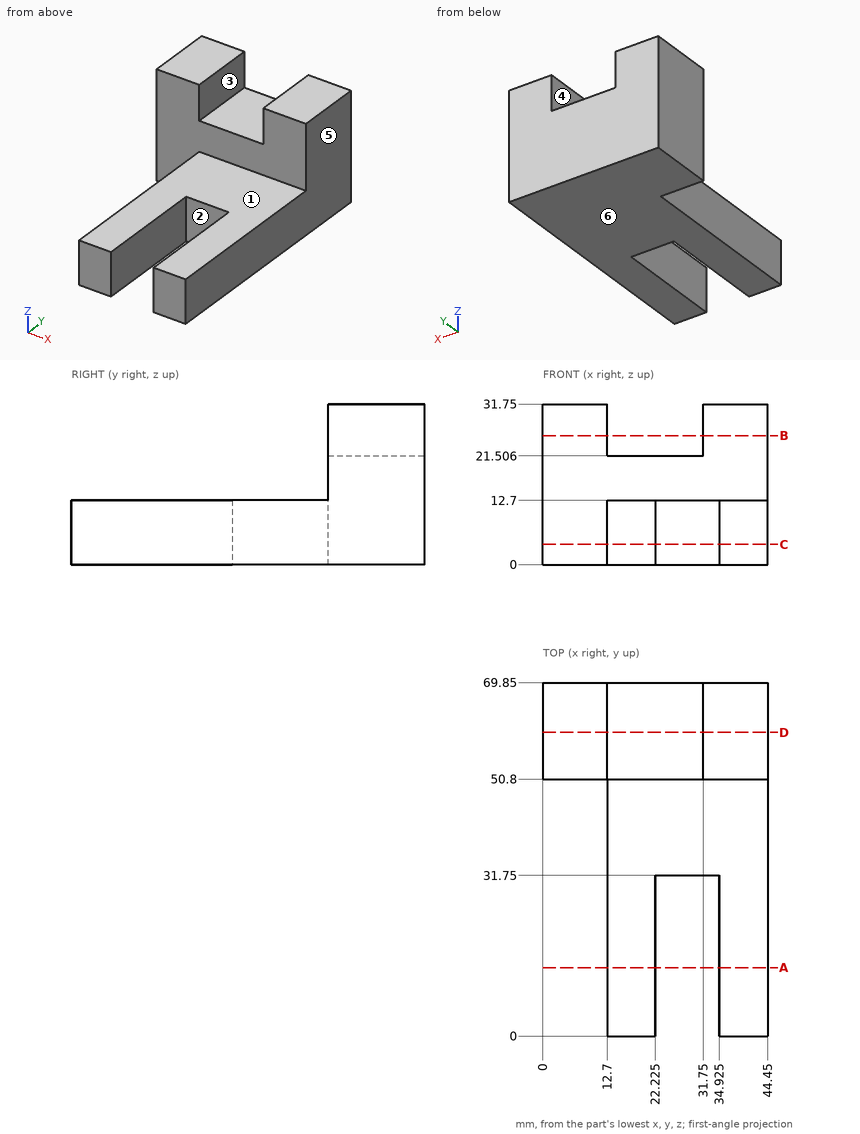
Print and shaded views of the part. All mm, measured from the part's lowest x, y and z. A direction names the side the tool comes from. Round coordinates to 2 decimals unless told otherwise and drop trailing zeros. Write each loop counter-clockwise with the first axis right and the second up, starting at its lowest first coordinate (ties: lowest second). Pieces come first, ordered by that corner, then holes. Notation, with made-up numbers: (55, 87.5) -> (110, 87.5) arc R10 ccw to (110, 106.5) -> close; hole circle Ø3 at (13, 3). An arc over 180 degrees is marked (long way). Answer in a Markdown table with one row per item. Add a question column.
Item 1: Saw through at D-D, the plane y = 60. Write the cut outline in (x, z).
Item 2: Saw through at A-A, the plane y = 13.5. Write the cut outline in (x, z) (3 decimals), then the cut area to 3 significant figures.
Item 3: Drop flat-ended pins along their axis: pin 1 Ø5 at (x, z) = (23, 20) entering from -Y; pin 2 Ø15 at (x, y) = (23, 65) entering from +Z; pin 3 Ø14 at (y, z) = (19, 3.5) entering from -X. Give the stop position or say it passes through.
Item 4: Drill centre lines: line 1 (X direction, y = 16, z = 9) (3 decimals); line 2 (X direction, y = 54, z = 23); line 3 (Y direction, x = 33, z = 22). Where is each one in solid material? Low to high. Write a range as from..to.
Item 5: Which spindle directions (+Z, -Z, +X, -X, +Y, -Y) get a long thin tool onto all of the face, cutting with end or side? Do the marked faces 1, 2 and 3. Say none if no direction does.
Item 6: Saw through at B-B, the plane z = 25.5. Write the cut outline in (x, y), then the cut area to 3 significant figures.
Item 7: Saw through at C-C, the plane z = 4. Write the cut outline in (x, y) (3 decimals).
Item 8: Mould opens along X. For the marked faces 4, 5 and 6 say: pulls with the +X half, pulls with the -X half, needs draft (parallel to the pull), parting line crosses it, or undercut.
Findings below:
| question | item | result |
|---|---|---|
| 1 | outline | (0, 0) -> (44.45, 0) -> (44.45, 31.75) -> (31.75, 31.75) -> (31.75, 21.51) -> (12.7, 21.51) -> (12.7, 31.75) -> (0, 31.75) -> close |
| 2 | outline | (12.7, 0) -> (22.225, 0) -> (22.225, 12.7) -> (12.7, 12.7) -> close; (34.925, 0) -> (44.45, 0) -> (44.45, 12.7) -> (34.925, 12.7) -> close |
| 2 | area | 242 mm^2 |
| 3 | pin 1 | stops at y = 50.8 |
| 3 | pin 2 | stops at z = 21.51 |
| 3 | pin 3 | stops at x = 12.7 |
| 4 | line 1 | x = 12.7..22.225, 34.925..44.45 |
| 4 | line 2 | x = 0..12.7, 31.75..44.45 |
| 4 | line 3 | y = 50.8..69.85 |
| 5 | face 1 | +Z, +X, -X, -Y |
| 5 | face 2 | +Z, -Z, -Y |
| 5 | face 3 | +Z, +Y, -Y |
| 6 | outline | (0, 50.8) -> (12.7, 50.8) -> (12.7, 69.85) -> (0, 69.85) -> close; (31.75, 50.8) -> (44.45, 50.8) -> (44.45, 69.85) -> (31.75, 69.85) -> close |
| 6 | area | 484 mm^2 |
| 7 | outline | (0, 50.8) -> (12.7, 50.8) -> (12.7, 0) -> (22.225, 0) -> (22.225, 31.75) -> (34.925, 31.75) -> (34.925, 0) -> (44.45, 0) -> (44.45, 69.85) -> (0, 69.85) -> close |
| 8 | face 4 | undercut |
| 8 | face 5 | pulls with the +X half |
| 8 | face 6 | needs draft |
